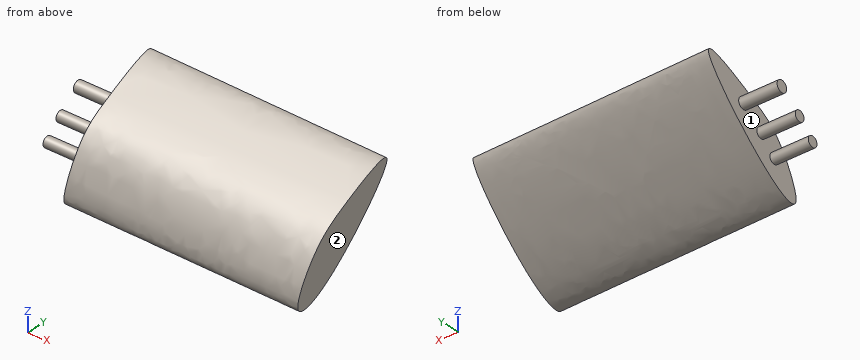
```python
from build123d import *

# Parameters (mm, degrees)
F4_R     = 3.7642677445
F4_R_2   = 3.4683059597
F4_R_3   = 3.4434090322
F5_DEPTH = 25.4


with BuildPart() as f3:
    # F2 (on offset) → F3 section 0
    with BuildSketch(Plane.YZ.offset(157.4308425188)):
        with BuildLine():
            add(Edge.make_bspline(
                [(0, 0), (-12.104644098, -6.3263168889), (-25.8820610041, -14.6136318994), (-47.8781855597, -52.5526708502), (-15.1609022465, -47.143178944), (53.8601710207, 26.7993739174), (11.9120155475, 6.2256423674), (0, 0)],
                knots=[0, 0, 0, 0, 0.1920446361, 0.3741659284, 0.5277277836, 0.8110114868, 1, 1, 1, 1], degree=3))
        make_face()
    # F0 (on Right) → F3 section 1
    with BuildSketch(Plane.YZ):
        with BuildLine():
            add(Edge.make_bspline(
                [(0, 0), (-11.4863605542, -5.9808116248), (-23.7079853047, -12.9240739578), (-43.9479848114, -53.9035395464), (-13.4752914458, -44.6437869025), (57.5158608034, 29.1418474769), (12.2926695837, 6.4006471675), (0, 0)],
                knots=[0, 0, 0, 0, 0.1834861231, 0.3694876095, 0.5199065669, 0.8036336859, 1, 1, 1, 1], degree=3))
        make_face()
    loft()

    # F4 (on face) → F5 (join)
    with BuildSketch(Plane(origin=(0, 0, 0), x_dir=(0, -1, 0), z_dir=(-1, 0, 0))):
        with Locations((-5.0992490724, -7.5565879233)):
            Circle(F4_R)
        with Locations((8.9653758332, -18.5892935842)):
            Circle(F4_R_2)
        with Locations((19.241169095, -28.9655476809)):
            Circle(F4_R_3)
    extrude(amount=F5_DEPTH)


solid = f3.part
```
Check sheet for the modelled part. Datum: model origin and axes. Units: mm. Face numbers are marked on the shaded views. A direction names the side the tool comes from. Give positions to 0.01 mm unless a question says otherwise; leave off trailing zeros. Answer as a JSON object with one key per item and string values. Group by question number.
1) Access from +Z, -Z, +X, -X, +Y, -Y to the whole of each face (thin tool, end or side, straight path). Record for the marked faces 1 and 2.
2) Depth check by flat-ended pin: P1, Ø12, axis at x = 106, y = -28.5, coming from the +Z side; P2, Ø10, axis at x = 11.5, y = -23, coming from the -Z side; P3, Ø12, axis at y = 0, z = -30, coming from the -X side. Enter the tip coordinate at first touch or a pass-through.
3) Thickness scan on probe 1 along X at (y, z) = (-24, -43); probe 2 along Z at (x, y) = (135.5, -9); probe 3 along Y at (x, z) = (139, -6). Record the ranges inside material, lowest first. Write a range as from..to.
Geometry results:
{
 "1": {"face 1": "-X", "face 2": "+Z, -Z, +X, +Y, -Y"},
 "2": {"P1": "stops at z = -15.38", "P2": "stops at z = -47.8", "P3": "stops at x = 0"},
 "3": {"probe 1": "x = 0..157.43", "probe 2": "z = -35.15..-4.91", "probe 3": "y = -10.81..20.97"}
}
